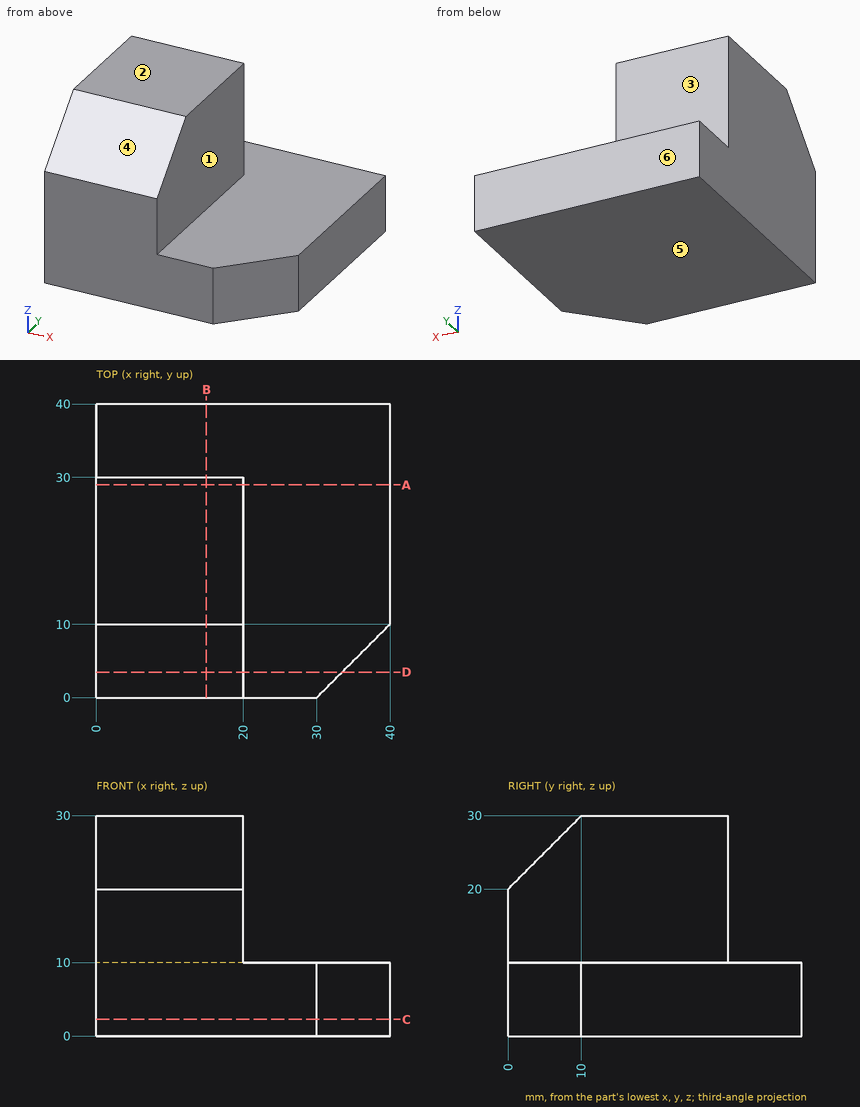
Geometry check sheet. Reference: drawing and pictorial views, mm from the part's lowest x, y, z. A direction names the side the tool comes from. Coordinates: 2 decimals unless noted, no trailing zeros. Loops run counter-clockwise (first coordinate to the right, second up) from the corner with the lowest first, then second, coordinate; pieces in that order, holes last. Notation, with made-up numbers: (-1.75, 52.25) - (33.25, 52.25) arc R22 cw to (33.25, 87.25) - close; hole circle Ø10 at (-26.5, 37). An arc over 180 degrees is marked (long way). Return JSON: item names as keys, results as strings.
1. Section check D-D, the plane y = 3.5. Record the boundary of the cut face in (x, z).
Established:
{"outline": "(0, 0) - (33.5, 0) - (33.5, 10) - (20, 10) - (20, 23.5) - (0, 23.5) - close"}
2. Section check C-C, the plane z = 2.25. Record the boundary of the cut face in (x, y).
Established:
{"outline": "(0, 0) - (30, 0) - (40, 10) - (40, 40) - (0, 40) - close"}
3. Thickness scan on L1, parallel to Y at x = 10.5, z = 15.5; L2, parallel to Z at x = 21, y = 9.5; L3, parallel to X at y = 4, z = 11. Record the ranges inside material, lowest first.
Established:
{"L1": "y = 0 to 30", "L2": "z = 0 to 10", "L3": "x = 0 to 20"}
4. Section check B-B, the plane x = 15. Record the boundary of the cut face in (y, z), then the cut area to 3 significant figures.
Established:
{"outline": "(0, 0) - (40, 0) - (40, 10) - (30, 10) - (30, 30) - (10, 30) - (0, 20) - close", "area": "950 mm2"}
5. Go/stop test with flat-tipped pins: pin 1 (4 mm diameter, centred on y = 21, z = 26, fed in from +X); pin 2 (8 mm diameter, centred on x = 21, z = 23, fed in from +Y). Record where each tip stops, or that it passes through.
Established:
{"pin 1": "stops at x = 20", "pin 2": "stops at y = 30"}
6. Section check A-A, the plane y = 29. Record the boundary of the cut face in (x, z), then the cut area to 3 significant figures.
Established:
{"outline": "(0, 0) - (40, 0) - (40, 10) - (20, 10) - (20, 30) - (0, 30) - close", "area": "800 mm2"}
7. Mould release check, pull along Z, two halves, no side actions. Record for the marked faces 4, 5 and 6: +Z half, -Z half, draft (parallel to the pull), parting line (faces both ways), or undercut.
Established:
{"face 4": "+Z half", "face 5": "-Z half", "face 6": "draft"}
8. Tool access check on the marked faces 1, 2 and 3. Record the directions out of +Z, -Z, +X, -X, +Y, -Y that give a thin tool (end or side, any length) a straight path to the whole face; none if there is none.
Established:
{"face 1": "+Z, +X, +Y, -Y", "face 2": "+Z, +X, -X, +Y, -Y", "face 3": "+Z, +X, -X, +Y"}
